Could you check a few things on this model? Use its own coordinates, in mm. Give positions to 0.01 mm unless a question says otherwise; leave off trailing zeros. Write each loop counter-clockwise with the first axis right and the second up, starting at its lowest first coordinate (ties: lowest second). Pieces come first, ordered by that corner, then holes. Notation, with made-up numbers: M 83.25,54 L 137.25,54 A17 cw 137.25,76 Z; hole C 43.25,13 d7. An arc over 180 degrees is marked long. One line per item, written item: value.
Autodesk Inventor part; units mm, degrees
ref_plane "YZ Plane" through (0, 0, 0) normal (1, 0, 0) x (0, 1, 0)
ref_plane "XZ Plane" through (0, 0, 0) normal (0, 1, 0) x (-1, 0, 0)
ref_plane "XY Plane" through (0, 0, 0) normal (0, 0, 1) x (1, 0, 0)
sketch "Sketch1" plane through (0, 0, 0) normal (0, 0, 1) x (1, 0, 0)
  circle A0 centre (0, 0) radius 2.0955
  circle A1 centre (91.581, 0) radius 2.0955
  circle A2 centre (0, 101.6) radius 2.0955
  circle A3 centre (91.581, 101.6) radius 2.0955
  line L0 (-6.35, -6.35) -> (92.075, -6.35)
  line L1 (98.425, 0) -> (98.425, 101.6)
  line L2 (92.075, 107.95) -> (-6.35, 107.95)
  line L3 (-6.35, 107.95) -> (-25.4396, 101.002)
  line L4 (-6.35, -6.35) -> (-25.4396, 0.598)
  line L5 (-6.35, -6.35) -> (13.9647, -6.35) construction
  line L6 (-42.1523, 24.4662) -> (-42.1523, 77.1338)
  arc A4 (-25.4396, 101.002) -> (-42.1523, 77.1338) centre (-16.7523, 77.1338) ccw
  arc A5 (-42.1523, 24.4662) -> (-25.4396, 0.598) centre (-16.7523, 24.4662) ccw
  arc A6 (98.425, 101.6) -> (92.075, 107.95) centre (92.075, 101.6) ccw
  arc A7 (92.075, -6.35) -> (98.425, 0) centre (92.075, 0) ccw
  circle A8 centre (92.075, 85.725) radius 2.0955
  circle A9 centre (92.075, 15.875) radius 2.0955
  point P0 (98.425, -6.35)
  point P1 (98.425, 107.95)
  point P2 (-42.1523, 94.919)
  point P3 (-42.1523, 6.681)
  dimension "d0" = 4.191
  dimension "d1" = 4.191
  dimension "d2" = 4.191
  dimension "d3" = 4.191
  dimension "d4" = 104.775
  dimension "d5" = 114.3
  dimension "d6" = 38.1
  dimension "d7" = 160
  dimension "d8" = 38.1
  dimension "d9" = 160
  dimension "d10" = 25.4
  dimension "d11" = 6.35
  dimension "d12" = 4.191
  dimension "d13" = 4.191
extrude "Extrusion1" add sketch "Sketch1" along normal blind 1.5875
properties part number "ramp" material "Acetal Resin, White"
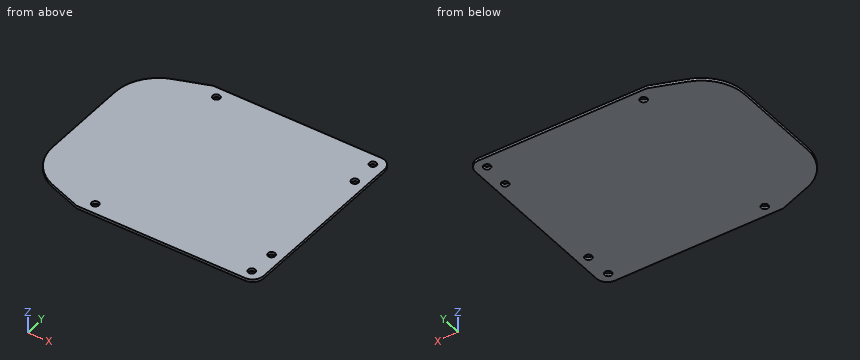
1) If we section it at A-A, the plane x = 0: Write out the boundary of the cut face in (y, z), then the cut area to 3 significant figures.
Outcome:
outline: M -6.35,0 L -2.1,0 L -2.1,1.59 L -6.35,1.59 Z; M 2.1,0 L 99.5,0 L 99.5,1.59 L 2.1,1.59 Z; M 103.7,0 L 107.95,0 L 107.95,1.59 L 103.7,1.59 Z
area: 168 mm^2
2) Please list where these lines run through material, in increasing order: L1, parallel to Y at x = 0, z = 0.75; L2, parallel to X at y = 85.5, z = 0.8 (3 decimals); L3, parallel to X at y = 83, z = 1.15 (3 decimals). Write a range as from..to.
Outcome:
L1: y = -6.35..-2.1, 2.1..99.5, 103.7..107.95
L2: x = -40.735..89.992, 94.158..98.425
L3: x = -41.466..98.425
3) I'm going to push a flat-ended pin straight in: pin 1 (3.5 mm diameter, centred on x = 91.581, y = 0, fed in from -Z). Where does the tip first touch, or does it pass through?
Outcome:
pin 1: passes through
4) If we section it at C-C, the plane y = 11: Write out the boundary of the cut face in (x, z) (1 decimal).
Outcome:
outline: M -38.3,0 L 98.4,0 L 98.4,1.6 L -38.3,1.6 Z
5) If we section it at B-B, the plane z = 0.4: Give the number of separate pieces and of enclosed holes in the cut face, then the cut area to 3 significant figures.
Outcome:
separate pieces: 1
enclosed holes: 6
area: 15,400 mm^2
